Here's how the part is built. I have some questions about the finished solid (model axes, mm). A direction names the side the tool comes from. Round coordinates to 2 decimals unless told otherwise and drop trailing zeros. Loops run counter-clockwise (first coordinate to the right, second up) from the corner with the lowest first, then second, coordinate; pieces in that order, holes last. Notation, with made-up numbers: (-23, 27.25) - (4, 27.25) arc R12 cw to (4, 38.25) - close; hole circle Ø3 at (5.5, 70). An arc over 180 degrees is marked (long way). Answer as a JSON object with one key per item and string values. Group by question number.
1) I want a section at A-A, the plane z = 3. Please give me the cut outline in (x, y).
2) I want a section at D-D, the plane y = -6. Please give me the cut outline in (x, z).
3) If I drill on line 1 along X through (y, z) = (-7.3, -30); line 2 along X through (y, z) = (16.15, 27.5); line 3 along Z through (x, y) = (3.75, -16), over which ranges is the centre line in solid material (lowest first)? Write a range as [from, to].
4) Which directions (+Z, -Z, +X, -X, +Y, -Y) give clear straight access to the entire face, cutting with the end or side of a thin tool? Please do faces 1 (the face through (-12, -12, 0)), 2 (the face through (18.14, -6.82, -15.54)), 3 (the face through (-2.334, -12.044, 25.494)), 4 (the face through (3.09, -14.81, -7.42)).
5) I want a section at B-B, the plane y = -16. Please give me the cut outline in (x, z), then the cut area to 3 significant figures.
6) I want a section at C-C, the plane x = 7. Please give me the cut outline in (y, z).
7) If we mould it in two halves opening along X, with no side actions, what happens to faces 5 (the face through (2, -12, -32)), 6 (the face through (2.85, 12.118, 5.345)), 7 (the face through (1.3, 16.479, 5.224))? For each: pulls with the +X half, pulls with the -X half, needs draft (parallel to the pull), parting line crosses it, or undercut.
8) Will these pins go through, and if not, where does the flat tip stop? P1, Ø1.4, axis at x = -6.25, z = -6.5, coming from the +Y side; P2, Ø1.3, axis at x = 13.5, z = -5.5, coming from the -Y side; P3, Ø0.9, axis at x = 3.75, z = -24, coming from the +Y side; P4, Ø0.9, axis at x = 1, z = 27.5, coming from the +Y side.
Autodesk Inventor part; units mm, degrees
ref_plane "YZ Plane" through (0, 0, 0) normal (1, 0, 0) x (0, 1, 0)
ref_plane "XZ Plane" through (0, 0, 0) normal (0, 1, 0) x (-1, 0, 0)
ref_plane "XY Plane" through (0, 0, 0) normal (0, 0, 1) x (1, 0, 0)
sketch "Sketch1" plane through (0, 0, 0) normal (0, 0, 1) x (1, 0, 0)
  line L0 (-15.5, 18) -> (19.5, 18)
  line L1 (19.5, 18) -> (19.5, -18)
  line L2 (19.5, -18) -> (-15.5, -18)
  line L3 (-15.5, -18) -> (-15.5, 18)
  point P0 (0, 0)
  dimension "d0" = 35
  dimension "d1" = 36
  dimension "d2" = 18
  dimension "d3" = 15.5
extrude "Extrusion1" add sketch "Sketch1" along normal blind 8
sketch "Sketch2" plane through (0, 0, 8) normal (0, 0, 1) x (1, 0, 0)
  line L0 (-15.5, 18) -> (19.5, 18)
  line L1 (19.5, 18) -> (19.5, -18)
  line L2 (19.5, -18) -> (-15.5, -18)
  line L3 (-15.5, -18) -> (-15.5, 18)
  line L4 (-15.5, -18) -> (-15.5, 18)
  line L5 (19.5, 18) -> (19.5, -18)
  line L6 (-15.5, 18) -> (19.5, 18)
  line L7 (19.5, -18) -> (-15.5, -18)
  line L8 (19.5, -18) -> (19.5, 18)
  point P0 (0, 0)
  dimension "d70" = 0
  dimension "d165" = 0
extrude "Extrusion2" add sketch "Sketch2" along normal blind 22.5
sketch "Sketch3" plane through (-15.5, -18, 0) normal (0, -1, 0) x (1, 0, 0)
  line L0 (7.85, 30.5) -> (7.35, 30.5)
  line L1 (7.85, 30.5) -> (8.35, 30.5)
  line L2 (35, 0) -> (0, 0)
  arc A0 (7.35, 20.7234) -> (8.35, 20.7234) centre (7.85, 16) ccw
  line L3 (7.35, 30.5) -> (7.35, 20.7234)
  line L4 (8.35, 30.5) -> (8.35, 20.7234)
  line L5 (35, 0) -> (35, 30.5)
  line L6 (35, 30.5) -> (0, 30.5)
  line L7 (0, 0) -> (0, 30.5)
  point P0 (15.5, 0)
  dimension "d16" = 0.5
  dimension "d17" = 0.5
  dimension "d63" = 9.4996
  dimension "d65" = 16
  dimension "d105" = 1
  dimension "d188" = 7.85
  dimension "d189" = 0.5
emboss "Emboss1" sketch "Sketch3" operation cut depth 50 direction (0, 1, 0) contours L1 L4 A0 L3 L0
sketch "Sketch13" plane through (0, 0, 0) normal (0, 0, -1) x (-1, 0, 0)
  line L0 (-13, -5.3) -> (11, -5.3)
  line L1 (15.5, 18) -> (-19.5, 18)
  line L2 (-19.5, 18) -> (-19.5, -18)
  line L3 (-19.5, -18) -> (15.5, -18)
  line L4 (15.5, -18) -> (15.5, 18)
  line L5 (-19.5, 18) -> (-19.5, -18)
  line L6 (-19.5, -5.3) -> (15.5, -5.3)
  point P0 (0, 0)
  dimension "d190" = 12.7
extrude "Extrusion5" add sketch "Sketch13" along normal blind 32 contours L0 L6 L4 L3 L2
sketch "Sketch14" plane through (-15.5, -5.3, 0) normal (0, 1, 0) x (1, 0, 0)
  line L0 (0, 32) -> (35, 32)
  line L1 (35, 0) -> (35, 32)
  point P0 (15.5, 0)
  point P1 (9.5, 30)
  point P2 (28, 30)
  point P3 (32.75, 16)
  dimension "d109" = 2
  dimension "d110" = 2
  dimension "d111" = 2.25
  dimension "d112" = 9.5
  dimension "d113" = 7
  dimension "d114" = 16
hole "Press fit for D2mm_L5mm Dowel - pin to protrude 2mm" at (-6, -5.3, -30) at (12.5, -5.3, -30) at (17.25, -5.3, -16) direction (0, -1, 0) diameter 2 depth 3 tip angle 118
sketch "Sketch21" plane through (0, 0, 0) normal (0, 0, -1) x (-1, 0, 0)
  circle A0 centre (-3.75, 0.2) radius 4
  circle A1 centre (-3.75, 0.2) radius 3 construction
  point P0 (0, 0)
  dimension "d185" = 8
extrude "Extrusion6" cut sketch "Sketch21" against normal through all
sketch "Sketch22" plane through (-15.5, -18, 30.5) normal (-1, 0, 0) x (0, 0, 1)
  line L0 (-30.5, 36) -> (0, 36)
  line L1 (-30.5, 12.7) -> (-30.5, 36)
  line L2 (-30.5, 12.7) -> (-62.5, 12.7)
  line L3 (-62.5, 0) -> (-62.5, 12.7)
  line L4 (0, 0) -> (-62.5, 0)
  line L5 (0, 0) -> (0, 36)
  point P0 (-30.5, 18)
  point P1 (-4, 30)
  point P2 (-4, 18)
  point P3 (-4, 6)
  dimension "d191" = 4
  dimension "d192" = 4
  dimension "d193" = 4
  dimension "d194" = 6
  dimension "d195" = 6
  dimension "d196" = 18
hole "CBore for M2.5 screw" [suppressed]
sketch "Sketch24" plane through (-7.65, -18, 16) normal (0, -1, 0) x (1, 0, 0)
  circle A0 centre (21.4, -42.5) radius 0.7835
  circle A1 centre (21.4, -22.5) radius 0.7835
  circle A2 centre (1.4, -42.5) radius 0.7835
  circle A3 centre (1.4, -22.5) radius 0.7835
  point P0 (7.65, -16)
hole "CBore for M2 screw" at (-6.25, -18, -6.5) at (13.75, -18, -6.5) at (13.75, -18, -26.5) at (-6.25, -18, -26.5) direction (0, 1, 0) diameter 2.4 end through all counterbore diameter 4.4 counterbore depth 5.2
sketch "Sketch25" plane through (-7.65, -18, 16) normal (0, -1, 0) x (1, 0, 0)
  circle A0 centre (21.4, -42.5) radius 2.2
  circle A1 centre (1.4, -22.5) radius 2.2
  circle A2 centre (21.4, -22.5) radius 2.2
  circle A3 centre (1.4, -42.5) radius 2.2
  line L0 (-0.5, 4.7234) -> (-0.5, 14.5)
  line L1 (-0.5, 14.5) -> (-7.85, 14.5)
  line L2 (-7.85, 14.5) -> (-7.85, -48)
  line L3 (27.15, -48) -> (-7.85, -48)
  line L4 (27.15, 14.5) -> (27.15, -48)
  line L5 (27.15, 14.5) -> (0.5, 14.5)
  line L6 (0.5, 14.5) -> (0.5, 4.7234)
  arc A4 (-0.5, 4.7234) -> (0.5, 4.7234) centre (0, 0) ccw
  line L7 (27.15, -48) -> (-7.85, -48)
  circle A5 centre (1.4, -42.5) radius 2.2
  circle A6 centre (21.4, -42.5) radius 1.2
  line L8 (1.4, -42.5) -> (21.4, -42.5) construction
  line L9 (11.4, -42.5) -> (11.4, 14.5) construction
  line L10 (0.5, 14.5) -> (27.15, 14.5)
  point P0 (7.65, -16)
  point P1 (11.4, -23)
  point P2 (11.4, -40)
  dimension "d218" = 8
  dimension "d219" = 25
hole "Threaded hole for M2 screw" at (3.75, -18, -7) at (3.75, -18, -24) direction (0, 1, 0) diameter 1.567 depth 6.3 tip angle 118
sketch "Sketch27" plane through (-15.5, 18, 0) normal (0, 1, 0) x (1, 0, 0)
  arc A0 (8.35, -20.7234) -> (7.35, -20.7234) centre (7.85, -16) ccw
  line L0 (7.35, -30.5) -> (7.35, -20.7234)
  arc A1 (8.35, -20.7234) -> (7.35, -20.7234) centre (7.85, -16) ccw
  line L1 (8.35, -20.7234) -> (8.35, -30.5)
  line L2 (8.35, -30.5) -> (35, -30.5)
  line L3 (35, 0) -> (35, -30.5)
  line L4 (0, 0) -> (35, 0)
  line L5 (0, 0) -> (0, -30.5)
  line L6 (0, -30.5) -> (7.35, -30.5)
  line L7 (7.85, -16) -> (7.85, -30.5)
  line L8 (7.85, -30.5) -> (0, -30.5)
  line L9 (0, -30.5) -> (0, 0)
  line L10 (0, 0) -> (7.85, 0)
  line L11 (7.85, 0) -> (7.85, -16)
  point P0 (15.5, 0)
extrude "Extrusion7" cut sketch "Sketch27" against normal through all contours L11 L7 L8 L0 A0 | A0 L0 L6 L5 L4 L11
sketch "Sketch23" plane through (-7.65, -18, 20.7234) normal (-1, 0, 0) x (0, 0, 1)
  line L0 (0, 0) -> (-9.4732, 0) construction
  line L1 (-9.4732, 36) -> (0, 36) construction
  line L2 (-4.7366, 0) -> (-4.7366, 36) construction
  point P0 (-20.7234, 18)
  point P1 (5.7766, 30)
  point P2 (5.7766, 18)
  point P3 (5.7766, 6)
  point P4 (-15.2498, 30)
  point P5 (-15.2498, 18)
  point P6 (-15.2498, 6)
  point P7 (5.7766, 30)
  point P8 (5.7766, 18)
  point P9 (5.7766, 6)
  dimension "d227" = 10.5132
  dimension "d228" = 10.5132
  dimension "d229" = 10.5132
  dimension "d230" = 10.5132
  dimension "d231" = 10.5132
  dimension "d232" = 10.5132
  dimension "d233" = 6
  dimension "d234" = 6
  dimension "d235" = 18
  dimension "d236" = 30
  dimension "d237" = 18
  dimension "d238" = 30
hole "Threaded hole for M2.5 screw" at (-7.65, 12, 26.5) at (-7.65, 0, 26.5) at (-7.65, -12, 26.5) at (-7.65, 12, 5.4736) at (-7.65, 0, 5.4736) at (-7.65, -12, 5.4736) direction (1, 0, 0) diameter 2.013 depth 10 tip angle 118
sketch "Sketch29" plane through (19.5, 18, 30.5) normal (0, 1, 0) x (1, 0, 0)
  arc A0 (-26.65, 9.7766) -> (-27.15, 19.2498) centre (-27.15, 14.5) ccw
  point P0 (-19.5, 30.5)
  point P1 (-23.5, 3)
  point P2 (-18.5, 3)
  point P3 (-23.5, 26)
  point P4 (-18.5, 26)
  dimension "d241" = 11.5
  dimension "d242" = 11.5
  dimension "d243" = 11.5
  dimension "d244" = 11.5
  dimension "d245" = 3.65
  dimension "d246" = 3.65
  dimension "d247" = 8.65
  dimension "d248" = 8.65
hole "Hole18" at (-4, 18, 27.5) at (1, 18, 27.5) at (-4, 18, 4.5) at (1, 18, 4.5) direction (0, -1, 0) diameter 1.567 depth 3 tip angle 118
equation "\"d2\" = 0.5 * d1"
properties part number "J007526" material "ALUMINUM, 6061-T651"
Outcome:
{
 "1": {"outline": "(-7.65, -18) - (19.5, -18) - (19.5, 18) - (-7.65, 18) - close; hole circle Ø8 at (3.75, 0.2)"},
 "2": {"outline": "(-15.5, -32) - (19.5, -32) - (19.5, 30.5) - (-7.15, 30.5) - (-7.15, 20.72) arc R4.75 cw to (-7.65, 11.25) - (-7.65, 0) - (-15.5, 0) - close; hole circle Ø2.4 at (-6.25, -26.5); hole circle Ø2.4 at (-6.25, -6.5); hole circle Ø2 at (-6, -30); hole circle Ø2 at (12.5, -30); hole circle Ø2.4 at (13.75, -26.5); hole circle Ø2.4 at (13.75, -6.5); hole circle Ø2 at (17.25, -16)"},
 "3": {"line 1": "[-15.5, -7], [-5, 11.5], [13.5, 19.5]", "line 2": "[-7.15, -4.78], [-3.22, 0.22], [1.78, 19.5]", "line 3": "[-32, -24.78], [-23.22, -7.78], [-6.22, 30.5]"},
 "4": {"face 1": "+Z, -X, +Y, -Y", "face 2": "+Y", "face 3": "-X", "face 4": "-Y"},
 "5": {"outline": "(-15.5, -32) - (19.5, -32) - (19.5, 30.5) - (-7.15, 30.5) - (-7.15, 20.72) arc R4.75 cw to (-7.65, 11.25) - (-7.65, 0) - (-15.5, 0) - close; hole circle Ø4.4 at (-6.25, -26.5); hole circle Ø4.4 at (-6.25, -6.5); hole circle Ø1.57 at (3.75, -24); hole circle Ø1.57 at (3.75, -7); hole circle Ø4.4 at (13.75, -26.5); hole circle Ø4.4 at (13.75, -6.5)", "area": "1,840 mm^2"},
 "6": {"outline": "(-18, -32) - (-5.3, -32) - (-5.3, 0) - (-2.13, 0) - (-2.13, 30.5) - (-18, 30.5) - close; (2.53, 0) - (18, 0) - (18, 30.5) - (2.53, 30.5) - close"},
 "7": {"face 5": "needs draft", "face 6": "pulls with the -X half", "face 7": "undercut"},
 "8": {"P1": "through", "P2": "y = -12.8", "P3": "y = -5.3", "P4": "y = 14.8"}
}
